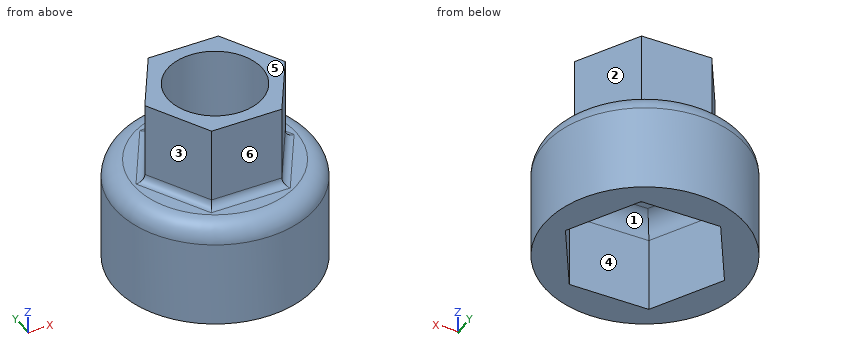
from build123d import *

# Parameters (mm, degrees)
SKETCH1_R           = 26.5
BOSS_EXTRUDE1_DEPTH = 25
SKETCH2_R           = 26.5
BOSS_EXTRUDE2_DEPTH = 25
CUT_EXTRUDE1_START  = -22
SKETCH3_R           = 26.5
CUT_EXTRUDE1_DEPTH  = 22
FILLET1_R           = 2
FILLET2_R           = 5
FILLET3_R           = 5
SKETCH4_R           = 12.5
CUT_EXTRUDE2_DEPTH  = 63.485998432


with BuildPart() as part:
    # Sketch1 → Boss-Extrude1 (new body)
    with BuildSketch(Plane.XY):
        Circle(SKETCH1_R)
        Polygon((10.421172359, 18.05), (-10.421172359, 18.05), (-20.842344718, 0), (-10.421172359, -18.05), (10.421172359, -18.05), (20.842344718, 0), align=None, mode=Mode.SUBTRACT)
    extrude(amount=BOSS_EXTRUDE1_DEPTH)

    # Sketch2 → Boss-Extrude2 (add)
    with BuildSketch(Plane.XY.offset(25)):
        Circle(SKETCH2_R)
    extrude(amount=BOSS_EXTRUDE2_DEPTH)

    # Sketch3 → Cut-Extrude1 (cut)
    with BuildSketch(Plane.XY.offset(50).offset(CUT_EXTRUDE1_START)):
        Circle(SKETCH3_R)
        Polygon((9.20178694, 15.937962501), (-9.20178694, 15.937962501), (-18.40357388, 0), (-9.20178694, -15.937962501), (9.20178694, -15.937962501), (18.40357388, 0), align=None, mode=Mode.SUBTRACT)
    extrude(amount=CUT_EXTRUDE1_DEPTH, mode=Mode.SUBTRACT)

    # Fillet1
    fillet1_edges = [part.edges().sort_by_distance(p)[0] for p in [
        (13.80268041, -7.96898125, 28),
        (13.80268041, 7.96898125, 28),
        (0, 15.937962501, 28),
        (-13.80268041, 7.96898125, 28),
        (-13.80268041, -7.96898125, 28),
        (0, -15.937962501, 28),
    ]]
    fillet(fillet1_edges, radius=FILLET1_R)

    # Fillet2
    fillet2_edges = [part.edges().sort_by_distance(p)[0] for p in [
        (15.631758538, 9.025, 25),
        (0, 18.05, 25),
        (-15.631758538, 9.025, 25),
        (-15.631758538, -9.025, 25),
        (0, -18.05, 25),
        (15.631758538, -9.025, 25),
    ]]
    fillet(fillet2_edges, radius=FILLET2_R)

    # Fillet3
    fillet3_edges = [part.edges().sort_by_distance(p)[0] for p in [
        (-26.5, 0, 28),
    ]]
    fillet(fillet3_edges, radius=FILLET3_R)

    # Sketch4 → Cut-Extrude2 (cut, through all)
    with BuildSketch(Plane.XY.offset(50)):
        Circle(SKETCH4_R)
    extrude(amount=-CUT_EXTRUDE2_DEPTH, mode=Mode.SUBTRACT)


solid = part.part
CAD build for the part. Positions are in the model's coordinates, mm. Face numbers are marked on the shaded views. A direction names the side the tool comes from. Coordinates: 2 decimals unless noted, no trailing zeros. Loops run counter-clockwise (first coordinate to the right, second up) from the corner with the lowest first, then second, coordinate; pieces in that order, holes last. Notation, with made-up numbers: (28, -17.5) -> (58, -17.5) arc R15 ccw to (58, 2.5) -> close; hole circle Ø2 at (48.5, -15). An arc over 180 degrees is marked (long way). One line per item, written item: value.
1. Slice it at B-B on x = 0. Write the cut outline in (y, z), and give its area (3 significant figures).
Answers:
outline: (-26.5, 0) -> (-18.05, 0) -> (-18.05, 20) arc R5 cw to (-13.05, 25) -> (-12.5, 25) -> (-12.5, 50) -> (-15.94, 50) -> (-15.94, 30) arc R2 cw to (-17.94, 28) -> (-21.5, 28) arc R5 ccw to (-26.5, 23) -> close; (12.5, 25) -> (13.05, 25) arc R5 cw to (18.05, 20) -> (18.05, 0) -> (26.5, 0) -> (26.5, 23) arc R5 ccw to (21.5, 28) -> (17.94, 28) arc R2 cw to (15.94, 30) -> (15.94, 50) -> (12.5, 50) -> close
area: 659 mm^2
2. Flat gauge pins, fed straight in: P1, Ø21, axis at x = -3.5, y = -6, coming from the -Z side; P2, Ø9, axis at x = 2, z = 38, coming from the +Y side; P3, Ø20, axis at x = -3, z = 40.5, coming from the -Y side; P4, Ø13, axis at x = 1.5, y = 2, coming from the +Z side. Where does each tip first touch, or does it go through?
Answers:
P1: stops at z = 23.59
P2: stops at y = 15.94
P3: stops at y = -15.94
P4: passes through
3. Which spindle directions (+Z, -Z, +X, -X, +Y, -Y) get a long thin tool onto all of the face, cutting with end or side? Do the marked faces 1, 2 and 3. Say none if no direction does.
Answers:
face 1: -Z
face 2: +Z, +X, +Y
face 3: +Z, -X, -Y
4. Slice it at C-C on z = 16.5. Write the cut outline in (x, y), and give its area (3 significant figures).
Answers:
outline: circle Ø53 at (0, 0); hole (-20.84, 0) -> (-10.42, -18.05) -> (10.42, -18.05) -> (20.84, 0) -> (10.42, 18.05) -> (-10.42, 18.05) -> close
area: 1,080 mm^2
5. Pull direction Y, two halves, no side cores. Call the marked faces 4, 5 and 6: pulls with the +Y half, pulls with the -Y half, needs draft (parallel to the pull), parting line crosses it, or undercut.
Answers:
face 4: undercut
face 5: needs draft
face 6: pulls with the -Y half
6. Drill centre lines: line 1 (Y direction, x = 0, z = 43); line 2 (Z direction, x = 14, y = -22); line 3 (X direction, y = -11.5, z = 36). Where is each one in solid material? Low to high. Write a range as [from, to].
Answers:
line 1: y = [-15.94, -12.5], [12.5, 15.94]
line 2: z = [0, 25.01]
line 3: x = [-11.76, -4.9], [4.9, 11.76]
7. Slice it at A-A on z = 33.5. Write the cut outline in (x, y), and give its area (3 significant figures).
Answers:
outline: (-18.4, 0) -> (-9.2, -15.94) -> (9.2, -15.94) -> (18.4, 0) -> (9.2, 15.94) -> (-9.2, 15.94) -> close; hole circle Ø25 at (0, 0)
area: 389 mm^2
